Part model, mm, in its own coordinate system. Face numbers are marked on the shaded views. Coordinates: 2 decimals unless noted, no trailing zeros. Write each loop counter-clockwise with the first axis right and the second up, starting at its lowest first coordinate (ties: lowest second). Pieces come first, ordered by that corner, then holes. Notation, with made-up numbers: (-13, 36.25) -> (1, 36.25) arc R30 ccw to (1, 66.25) -> close; hole circle Ø2 at (49.25, 74.25). An arc over 180 degrees is marked (long way). One line per question, with ' | ' between items. Start each with the question number.
Item 1: Two-plate mould, pull along Y, no slides. Class the marked faces 1, 2 and 3: pulls with the +Y half, pulls with the -Y half, needs draft (parallel to the pull), parting line crosses it, or undercut.
Item 2: Saw through at C-C (x = -25.5). Count the separate pieces of the cut face and the enclosed holes in it, and give its area (3 significant figures).
Item 3: Saw through at A-A (z = 14). List the corners of the cut face in (x, y), and give its area (3 significant figures).
Item 4: Pin check, flat tips, straight feed: pin 1 (2.5 mm diameter, centred on y = 4, z = -6.5, fed in from +X); pin 2 (17 mm diameter, centred on x = 11.5, z = -5.5, fed in from +Y); pin 3 (2 mm diameter, centred on y = 109.5, z = -1.5, fed in from -X). Stop position of each tip, or through.
Item 5: Saw through at B-B (y = 95). List the corners of the cut face in (x, z).
Item 6: Probe probe 1 along X at (y, z) = (119, 4); probe 2 along Z at (x, y) = (62.5, 77); probe 3 along X at (y, z) = (98, 5.5). List the from-to ranges inside material, lowest first. Write a range as [from, to].
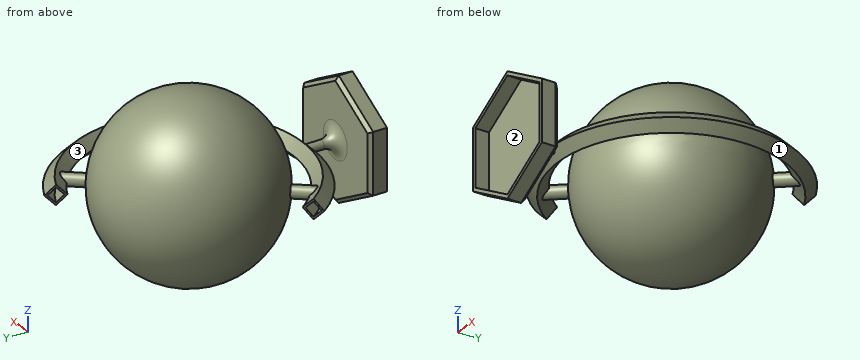
from build123d import *

# Parameters (mm, degrees)
BOSS_EXTRUDE1_DEPTH             = 10
SHELL1_T                        = -2
REVOLVE_THIN1_ANGLE             = 55
REVOLVE_THIN1_OTHER_WAY_ANGLE   = 155
BOSS_EXTRUDE2_REACH             = 157.311
SKETCH5_R                       = 3.5
BOSS_EXTRUDE2_DIRECTION_2_REACH = 157.311
BOSS_EXTRUDE3_REACH             = 174.35
SKETCH6_R                       = 2.5
FILLET1_R                       = 8
CHAMFER1_SIZE                   = 2


with BuildPart() as part:
    # Sketch1 → Boss-Extrude1 (new body)
    with BuildSketch(Plane(origin=(0, 0, 0), x_dir=(1, 0, 0), z_dir=(0, 1, 0))):
        Polygon((0, 35), (-30.310889132, 17.5), (-30.310889132, -17.5), (0, -35), (30.310889132, -17.5), (30.310889132, 17.5), align=None)
    extrude(amount=BOSS_EXTRUDE1_DEPTH)

    # Shell1
    shell1_openings = [part.faces().sort_by_distance(p)[0] for p in [
        (0, 0, 0),
    ]]
    offset(amount=SHELL1_T, openings=shell1_openings, kind=Kind.INTERSECTION)


with BuildPart() as body_2:
    # Sketch2 → Revolve1 (revolve)
    with BuildSketch(Plane.XY):
        with BuildLine():
            Line((0, 145), (0, 45))
            ThreePointArc((0, 45), (50, 95), (0, 145))
        make_face()
    revolve(axis=Axis((0, 145, 0), (0, -1, 0)))


with BuildPart() as body_3:
    # Sketch4 → Revolve-Thin1 (revolve)
    with BuildSketch(Plane(origin=(0, 0, 0), x_dir=(0, 0, -1), z_dir=(1, 0, 0))):
        Polygon((0, 24.343145751), (-5.656854249, 30), (0, 35.656854249), (5.656854249, 30), align=None)
        Polygon((0, 25.757359313), (-4.242640687, 30), (0, 34.242640687), (4.242640687, 30), align=None, mode=Mode.SUBTRACT)
    revolve(axis=Axis((0, 95, 0), (0, 0, -1)), revolution_arc=REVOLVE_THIN1_ANGLE)

    # Sketch4 → Revolve-Thin1 other way (revolve)
    with BuildSketch(Plane(origin=(0, 0, 0), x_dir=(0, 0, -1), z_dir=(1, 0, 0))):
        Polygon((0, 24.343145751), (-5.656854249, 30), (0, 35.656854249), (5.656854249, 30), align=None)
        Polygon((0, 25.757359313), (-4.242640687, 30), (0, 34.242640687), (4.242640687, 30), align=None, mode=Mode.SUBTRACT)
    revolve(axis=Axis((0, 95, 0), (0, 0, 1)), revolution_arc=REVOLVE_THIN1_OTHER_WAY_ANGLE)

    # Sketch5 → Boss-Extrude2 (add, up to next)
    with BuildSketch(Plane(origin=(46.778368268, 55.748288439, 0), x_dir=(0, 0, 1), z_dir=(0.6427876096865406, 0.7660444431189771, 0)), mode=Mode.PRIVATE) as boss_extrude2_sk1:
        with Locations(Location((0, -61.06482292, 0), (0, 0, 89.999995384))):
            Circle(SKETCH5_R)
    boss_extrude2_tool1 = extrude(boss_extrude2_sk1.sketch, amount=BOSS_EXTRUDE2_REACH, mode=Mode.PRIVATE) - body_3.part

    add(body_2.part)  # Boss-Extrude2 merges body 2
    add(boss_extrude2_tool1.solids().sort_by_distance((0, 95, 0))[0])

    # Sketch5 → Boss-Extrude2 direction 2 (add, up to next)
    with BuildSketch(Plane(origin=(46.778368268, 55.748288439, 0), x_dir=(0, 0, 1), z_dir=(0.6427876096865406, 0.7660444431189771, 0)), mode=Mode.PRIVATE) as boss_extrude2_direction_2_sk1:
        with Locations(Location((0, -61.06482292, 0), (0, 0, 89.999995384))):
            Circle(SKETCH5_R)
    boss_extrude2_direction_2_tool1 = extrude(boss_extrude2_direction_2_sk1.sketch, amount=-BOSS_EXTRUDE2_DIRECTION_2_REACH, mode=Mode.PRIVATE) - body_3.part
    add(boss_extrude2_direction_2_tool1.solids().sort_by_distance((0, 95, 0))[0])

    # Sketch6 → Boss-Extrude3 (add, up to next)
    with BuildSketch(Plane(origin=(0, 10, 0), x_dir=(1, 0, 0), z_dir=(0, 1, 0)), mode=Mode.PRIVATE) as boss_extrude3_sk1:
        with Locations(Location((0, 0, 0), (0, 0, 179.999998803))):
            Circle(SKETCH6_R)
    boss_extrude3_tool1 = extrude(boss_extrude3_sk1.sketch, amount=BOSS_EXTRUDE3_REACH, mode=Mode.PRIVATE) - body_3.part

    add(part.part)  # Boss-Extrude3 merges part
    add(boss_extrude3_tool1.solids().sort_by_distance((0, 10, 0))[0])

    # Fillet1
    fillet1_edges = [body_3.edges().sort_by_distance(p)[0] for p in [
        (2.5, 10, 5.2e-08),
    ]]
    fillet(fillet1_edges, radius=FILLET1_R)

    # Chamfer1
    chamfer1_edges = [body_3.edges().sort_by_distance(p)[0] for p in [
        (-30.310889132, 10, 0),
        (-15.155444566, 10, 26.25),
        (15.155444566, 10, 26.25),
        (30.310889132, 10, 0),
        (15.155444566, 10, -26.25),
        (-15.155444566, 10, -26.25),
    ]]
    chamfer(chamfer1_edges, length=CHAMFER1_SIZE)


solid = body_3.part
From the geometry:
1) face 1: undercut | face 2: pulls with the -Y half | face 3: undercut
2) separate pieces: 3 | enclosed holes: 1 | area: 5,960 mm2
3) outline: circle Ø96 at (0, 95); (-30.31, 0) -> (-28.31, 0) -> (-28.31, 8) -> (28.31, 8) -> (28.31, 0) -> (30.31, 0) -> (30.31, 8) -> (28.31, 10) -> (-28.31, 10) -> (-30.31, 8) -> close | area: 7,390 mm2
4) pin 1: x = 30.31 | pin 2: y = 144.82 | pin 3: x = -48.12
5) outline: circle Ø100 at (0, 0); (59.34, 0) -> (65, -5.66) -> (70.66, 0) -> (65, 5.66) -> close; hole (60.76, 0) -> (65, -4.24) -> (69.24, 0) -> (65, 4.24) -> close
6) probe 1: [-43.68, 43.68], [58.62, 60.15], [60.67, 62.19] | probe 2: [-5.62, -4.2], [4.2, 5.62] | probe 3: [-49.61, 49.61], [64.77, 65.09]
